Design review of the part shown in the three views and the two pictorial views. Dimensions are in mm from the part's minimum x, y and z. A direction names the side the tool comes from. Give positions to 0.01 mm unless a question says otherwise; leave off trailing zeros. Order: outer loops, then holes, each group sorted by start corner. A loop starts at its lowest first (then second) coordinate and runs counter-clockwise, first axis right, second up.
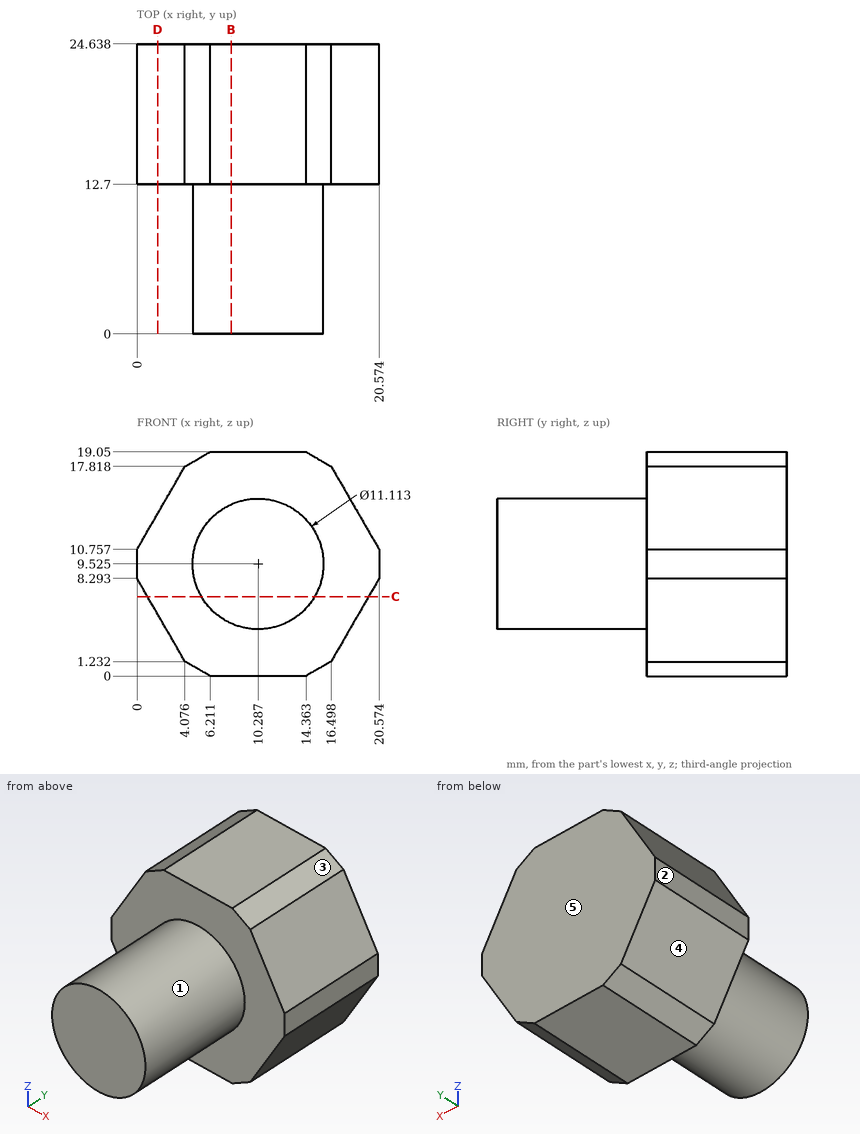
1) To check wall thickness, follow line 1 (Z direction, x = 2.5, y = 21) (1 decimal); line 2 (Y direction, x = 7.5, z = 4); line 3 (X direction, y = 4.25, z = 13.5) (1 decimal). State the ranges of each line that lie inside material, in increasing order.
Answer sheet:
line 1: z = 4 to 15.1
line 2: y = 12.7 to 24.64
line 3: x = 6.4 to 14.2
2) We need section D-D on x = 1.75. Give the boundary of the cut face in (y, z).
Answer sheet:
outline: (12.7, 5.26) - (24.64, 5.26) - (24.64, 13.79) - (12.7, 13.79) - close
3) We need section B-B on x = 8. Give the boundary of the cut face in (y, z).
Answer sheet:
outline: (0, 4.46) - (12.7, 4.46) - (12.7, 0) - (24.64, 0) - (24.64, 19.05) - (12.7, 19.05) - (12.7, 14.59) - (0, 14.59) - close
4) Clearance check with flat-ended pins moving along their axes: pin 1 (1 mm diameter, centred on y = 16.5, z = 7, fed in from -X); pin 2 (4 mm diameter, centred on y = 6.5, z = 6, fed in from +X); pin 3 (6 mm diameter, centred on y = 8.5, z = 3.5, fed in from +X). State where each tip first meets the part, or that it passes through.
Answer sheet:
pin 1: stops at x = 0.46
pin 2: stops at x = 15.63
pin 3: stops at x = 14.95
5) Draft analysis for pull direction Z (two halves, no side actions). For the marked faces 3, 4 and 5, state which applies: +Z half, -Z half, draft (parallel to the pull), parting line (faces both ways), or undercut.
Answer sheet:
face 3: +Z half
face 4: -Z half
face 5: draft
6) Tool access review of the marked faces 1 and 2: name each direction out of +Z, -Z, +X, -X, +Y, -Y from which nothing blocks a thin tool from reaching the whole face with its end or side.
Answer sheet:
face 1: -Y
face 2: +Z, -Z, -X, +Y, -Y
7) We need section C-C on z = 6.75. Give the boundary of the cut face in (x, y).
Answer sheet:
outline: (0.89, 12.7) - (5.47, 12.7) - (5.47, 0) - (15.1, 0) - (15.1, 12.7) - (19.68, 12.7) - (19.68, 24.64) - (0.89, 24.64) - close
